```python
from build123d import *

# Parameters (mm, degrees)
ESQUISSE1_R             = 115
ESQUISSE1_R_2           = 22.5
BOSS_EXTRU_1_DEPTH      = 6
ENL_V_MAT_EXTRU_2_DEPTH = 6


with BuildPart() as part:
    # Esquisse1 → Boss.-Extru.1 (new body)
    with BuildSketch(Plane.XY):
        Circle(ESQUISSE1_R)
        Circle(ESQUISSE1_R_2, mode=Mode.SUBTRACT)
    extrude(amount=BOSS_EXTRU_1_DEPTH)

    # Esquisse2 → Enlèv. mat.-Extru.2 (cut)
    with BuildSketch(Plane.XY.offset(6)):
        Polygon((-114.755174175, 7.5), (-99.755174175, 7.5), (-99.755174175, -7.5), (-114.755174175, -7.5), (-126.610711634, 0), align=None)
    extrude(amount=-ENL_V_MAT_EXTRU_2_DEPTH, mode=Mode.SUBTRACT)


solid = part.part
```
Check sheet for the modelled part. Datum: model origin and axes. Units: mm. A direction names the side the tool comes from. Round coordinates to 2 decimals unless told otherwise and drop trailing zeros. Loops run counter-clockwise (first coordinate to the right, second up) from the corner with the lowest first, then second, coordinate; pieces in that order, holes last. Notation, with made-up numbers: M -14,-17.75 L 23,-17.75 A26 ccw 23,19.25 Z; hole C -33.5,22 d7. An arc over 180 degrees is marked long. Answer as a JSON object with one key per item and string values.
1. Section check B-B (z = 4.35). Record the boundary of the cut face in (x, y).
Reply:
{"outline": "M -114.76,-7.5 A115 ccw long -114.76,7.5 L -99.76,7.5 L -99.76,-7.5 Z; hole C 0,0 d45"}
2. Section check C-C (y = -48.5). Record the boundary of the cut face in (x, z), plus the area to 3 significant figures.
Reply:
{"outline": "M -104.27,0 L 104.27,0 L 104.27,6 L -104.27,6 Z", "area": "1,250 mm²"}
3. Mould release check, pull along Y, two halves, no side actions. Record for faces 1 (the flat face through (-107, 7.5, 3)), 2 (the flat face through (-1, -24, 0)), 3 (the cylindrical face through (10.382, -19.961, 2.958)): pulls with the +Y half, pulls with the -Y half, needs draft (parallel to the pull), parting line crosses it, or undercut.
Reply:
{"face 1": "undercut", "face 2": "needs draft", "face 3": "undercut"}
4. Gauge pin test, flat ends, axial feed: P1, Ø5, axis at x = 27.5, y = 32.5, coming from the -Z side; P2, Ø3, axis at y = 2, z = 4, coming from the -X side; P3, Ø3, axis at x = -68.5, z = 4, coming from the -Y side; P4, Ø1.8, axis at x = -104.5, z = 2, coming from the -Y side. Record the tip position at first contact, or that the pin passes through.
Reply:
{"P1": "stops at z = 0", "P2": "stops at x = -99.76", "P3": "stops at y = -93.47", "P4": "stops at y = -49.92"}
5. Access from +Z, -Z, +X, -X, +Y, -Y to the whole of each face (thin tool, end or side, straight path). Record for faces 4 (the flat face through (-1, -24, 6)), 5 (the flat face through (-99.755, 0, 3)).
Reply:
{"face 4": "+Z, +X, -X, +Y, -Y", "face 5": "+Z, -Z, -X"}
6. Section check D-D (x = 51). Record the boundary of the cut face in (y, z).
Reply:
{"outline": "M -103.07,0 L 103.07,0 L 103.07,6 L -103.07,6 Z"}
7. Section check A-A (x = 0). Record the boundary of the cut face in (y, z), plus the area to 3 significant figures.
Reply:
{"outline": "M -115,0 L -22.5,0 L -22.5,6 L -115,6 Z; M 22.5,0 L 115,0 L 115,6 L 22.5,6 Z", "area": "1,110 mm²"}
8. Scan lines: line 1 (Y direction, x = 0, z = 3.1); line 2 (X direction, y = -11.5, z = 3.05); line 3 (Y direction, x = -14.5, z = 2.7). Record each from-to range of solid material in increasing order.
Reply:
{"line 1": "y = -115 to -22.5, 22.5 to 115", "line 2": "x = -114.42 to -19.34, 19.34 to 114.42", "line 3": "y = -114.08 to -17.2, 17.2 to 114.08"}
